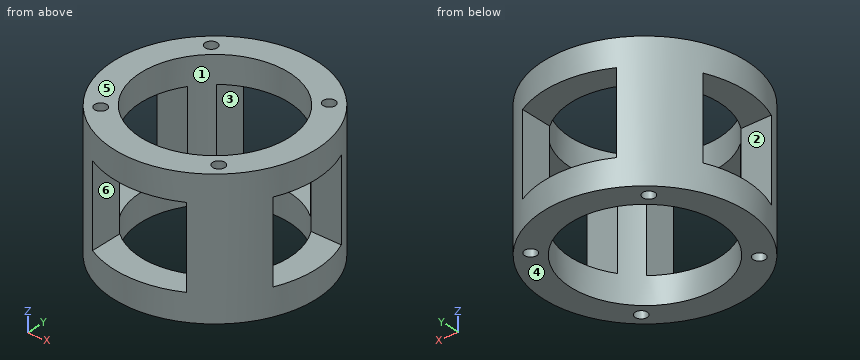
from build123d import *

# Parameters (mm, degrees)
F0_R          = 37.5
F0_R_2        = 27.5
F2_DEPTH      = 50
F3_W          = 35
F3_H          = 30
F4_DEPTH      = 37.501
F4_DEPTH_BACK = 37.501
F5_W          = 30
F5_H          = 30
F6_DEPTH      = 37.501
F6_DEPTH_BACK = 37.501
F8_D          = 4.5
F8_DEPTH      = 6
F8_TIP        = 1.3519363928
F10_D         = 4.5
F10_DEPTH     = 6
F10_TIP       = 1.3519363928


with BuildPart() as f2:
    # F0 (on Top) → F2 (new body)
    with BuildSketch(Plane.XY):
        Circle(F0_R)
        Circle(F0_R_2, mode=Mode.SUBTRACT)
    extrude(amount=F2_DEPTH)

    # F3 (on Front) → F4 (cut, two sides)
    with BuildSketch(Plane.XZ) as f4_sk:
        with Locations((0, 25)):
            Rectangle(F3_W, F3_H)
    extrude(amount=-F4_DEPTH, mode=Mode.SUBTRACT)
    extrude(f4_sk.sketch, amount=F4_DEPTH_BACK, mode=Mode.SUBTRACT)

    # F5 (on Right) → F6 (cut, two sides)
    with BuildSketch(Plane.YZ) as f6_sk:
        with Locations((0, 25)):
            Rectangle(F5_W, F5_H)
    extrude(amount=-F6_DEPTH, mode=Mode.SUBTRACT)
    extrude(f6_sk.sketch, amount=F6_DEPTH_BACK, mode=Mode.SUBTRACT)

    # F8
    with Locations(Plane.XY.offset(50)):
        with Locations((21.8730719462, -24.0378602133), (24.0378602133, 21.8730719462), (-21.8730719462, 24.0378602133), (-24.0378602133, -21.8730719462)):
            Hole(F8_D / 2, depth=F8_DEPTH)
            with Locations((0, 0, -(F8_DEPTH + F8_TIP / 2))):  # 118° drill point
                Cone(0, F8_D / 2, F8_TIP, mode=Mode.SUBTRACT)

    # F10
    with Locations(Plane(origin=(0, 0, 0), x_dir=(1, 0, 0), z_dir=(0, 0, -1))):
        with Locations((21.8730719462, 24.0378602133), (24.0378602133, -21.8730719462), (-24.0378602133, 21.8730719462), (-21.8730719462, -24.0378602133)):
            Hole(F10_D / 2, depth=F10_DEPTH)
            with Locations((0, 0, -(F10_DEPTH + F10_TIP / 2))):  # 118° drill point
                Cone(0, F10_D / 2, F10_TIP, mode=Mode.SUBTRACT)


solid = f2.part
The model under review builds one solid part; all positions refer to its coordinate system, in mm. Face numbers are marked on the shaded views. A direction names the side the tool comes from. Round coordinates to 2 decimals unless told otherwise and drop trailing zeros. Write each loop counter-clockwise with the first axis right and the second up, starting at its lowest first coordinate (ties: lowest second). Pieces come first, ordered by that corner, then holes. Notation, with made-up numbers: M 63,55 L 90,55 A20 cw 90,73 Z; hole C 45.25,-29.75 d4. An arc over 180 degrees is marked long. Use a Markdown table: item, result. Add a question column.
Q1. We need section B-B, the plane y = 0. State the section outline as (x, z) points, plus the area to 3 significant figures.
Q2. To check wall thickness, follow line 1 (Z direction, x = 26, y = -13); line 2 (X direction, y = -17.5, z = 40); line 3 (X direction, y = -21, z = 3.5). State the ranges of each line that lie inside material, in increasing order.
Q3. We need section C-C, the plane y = 17. State the section outline as (x, z) points, plus the area to 3 significant figures.
Q4. Insertion check: pin 1 (4 mm diameter, centred on x = -21.87, y = 24.04, fed in from +Z); pin 2 (5 mm diameter, centred on x = -19.5, z = 30.5, fed in from +Y); pin 3 (10 mm diameter, centred on y = 17, z = 41.5, fed in from +X). Each pin has a flat end and moves straight along its axis. Give the tip position at first contact, or say it passes through.
Q5. We need section A-A, the plane x = -15. State the section outline as (y, z) points, plus the area to 3 significant figures.
Q6. The part is to be moulded in two halves that separate along Z. For the marked faces 4, 5 and 6, say which applies: pulls with the +Z half, pulls with the -Z half, needs draft (parallel to the pull), parting line crosses it, or undercut.
Q7. Machinability: for the marked faces 1, 2 and 3, which of the approach directions +Z, -Z, +X, -X, +Y, -Y give a long, thin tool a straight path to every point of the face, cutting with its end or side? Answer none if there is none.
Findings below:
| question | item | result |
|---|---|---|
| 1 | outline | M -37.5,0 L -27.5,0 L -27.5,10 L -37.5,10 Z; M -37.5,40 L -27.5,40 L -27.5,50 L -37.5,50 Z; M 27.5,0 L 37.5,0 L 37.5,10 L 27.5,10 Z; M 27.5,40 L 37.5,40 L 37.5,50 L 27.5,50 Z |
| 1 | area | 400 mm² |
| 2 | line 1 | z = 0 to 10, 40 to 50 |
| 2 | line 2 | x = -33.17 to -21.21, 21.21 to 33.17 |
| 2 | line 3 | x = -31.07 to -26.11, -21.96 to -17.76, 17.76 to 31.07 |
| 3 | outline | M -33.43,0 L -21.62,0 L -21.62,50 L -33.43,50 Z; M 21.62,0 L 33.43,0 L 33.43,50 L 21.62,50 Z |
| 3 | area | 1,180 mm² |
| 4 | pin 1 | stops at z = 43.85 |
| 4 | pin 2 | stops at y = 33.17 |
| 4 | pin 3 | stops at x = 35.53 |
| 5 | outline | M -34.37,0 L -23.05,0 L -23.05,10 L -34.37,10 Z; M -34.37,40 L -23.05,40 L -23.05,50 L -34.37,50 Z; M 23.05,0 L 34.37,0 L 34.37,10 L 23.05,10 Z; M 23.05,40 L 34.37,40 L 34.37,50 L 23.05,50 Z |
| 5 | area | 453 mm² |
| 6 | face 4 | pulls with the -Z half |
| 6 | face 5 | pulls with the +Z half |
| 6 | face 6 | undercut |
| 7 | face 1 | +Z, -Z |
| 7 | face 2 | +X, -X |
| 7 | face 3 | +Y, -Y |
